Autodesk Inventor part; units mm, degrees
ref_plane "YZ Plane" through (0, 0, 0) normal (1, 0, 0) x (0, 1, 0)
ref_plane "XZ Plane" through (0, 0, 0) normal (0, 1, 0) x (-1, 0, 0)
ref_plane "XY Plane" through (0, 0, 0) normal (0, 0, 1) x (1, 0, 0)
sketch "Sketch1" plane through (0, 0, 0) normal (0, 0, 1) x (1, 0, 0)
  line L0 (-4.5718, -2.6632) -> (-7.5718, -2.6632)
  line L1 (-7.5718, -2.6632) -> (-7.5718, -10.8132)
  line L2 (-7.5718, -10.8132) -> (-4.5718, -10.8132)
  line L3 (-4.5718, -10.8132) -> (-4.5718, -2.6632)
  dimension "d1" = 8.15
  dimension "d2" = 3
revolve "Shoulder" add sketch "Sketch1" angle 360 about axis through (-4.5718, -10.8132, 0) along (0, 1, 0)
sketch "Sketch2" plane through (-4.5718, -2.6632, 0) normal (0, 1, 0) x (1, 0, 0)
  circle A0 centre (0, 0) radius 3
  circle A1 centre (0, 0) radius 2.76
  dimension "d3" = 5.52
extrude "Shoulder_neck" add sketch "Sketch2" along normal blind 1.85 contours A1
sketch "Sketch3" plane through (-4.5718, -0.8132, 0) normal (0, 1, 0) x (1, 0, 0)
  circle A0 centre (0, 0) radius 2.76
  circle A1 centre (0, 0) radius 5.075
  dimension "d6" = 10.15
extrude "Head" add sketch "Sketch3" along normal blind 4.5 contours A0 | A1
sketch "Sketch4" plane through (-4.5718, -10.8132, 0) normal (0, -1, 0) x (1, 0, 0)
  circle A0 centre (0, 0) radius 3
  circle A1 centre (0, 0) radius 1.89
  dimension "d9" = 3.78
extrude "Thread_neck" add sketch "Sketch4" along normal blind 1.8 contours A1
sketch "Sketch5" plane through (-4.5718, -12.6132, 0) normal (0, -1, 0) x (1, 0, 0)
  circle A0 centre (0, 0) radius 1.89
  circle A1 centre (0, 0) radius 2.5
  dimension "d12" = 5
extrude "Thread_shoulder" add sketch "Sketch5" along normal blind 7.7 contours A0 | A1
sketch "Sketch6" plane through (-4.5718, 3.6868, 0) normal (0, 1, 0) x (1, 0, 0)
  circle A0 centre (0, 0) radius 5.075
  circle A1 centre (0, 0) radius 1.5 construction
  line L0 (-1.5, 0.866) -> (-1.5, -0.866)
  line L1 (-1.5, -0.866) -> (0, -1.7321)
  line L2 (0, -1.7321) -> (1.5, -0.866)
  line L3 (1.5, -0.866) -> (1.5, 0.866)
  line L4 (1.5, 0.866) -> (0, 1.7321)
  line L5 (0, 1.7321) -> (-1.5, 0.866)
  dimension "d15" = 3
extrude "Hex" cut sketch "Sketch6" against normal blind 2.4 contours L5 L4 L3 L2 L1 L0
chamfer "Chamfer1" distance 0.24 angle 30 1 edges at (-1.5718, -2.6632, 0) measured on face at (-7.436, -2.6632, -0.4595)
fillet "Fillet1" radius 0.4 1 edges at (-7.3318, -0.8132, 0)
chamfer "Chamfer2" distance 0.3 angle 30 1 edges at (-9.6468, 3.6868, 0) measured on face at (0.4867, 2.1868, 0.4084)
chamfer "Chamfer3" distance 0.4 angle 30 1 edges at (-7.0718, -20.3132, 0) measured on face at (-3.3106, -20.3132, -0.6619)
fillet "Fillet2" radius 0.6 1 edges at (-6.4618, -10.8132, 0)
chamfer "Chamfer7" distance 0.61 angle 30 1 edges at (-7.0718, -12.6132, 0) measured on face at (-2.3177, -12.6132, -0.3502)
thread "Thread"
equation "\"d1\" = Shoulder_length - Shoulder_neck_length"
equation "\"d2\" = 0.5 * Shoulder_diameter"
equation "\"d3\" = Shoulder_neck_dia"
equation "\"d4\" = Shoulder_neck_length"
equation "\"d6\" = Head_diameter"
equation "\"d7\" = Head_height"
equation "\"d9\" = Thread_neck_dia"
equation "\"d10\" = Thread_neck_length"
equation "\"d12\" = Thread_diameter"
equation "\"d13\" = Thread_length - Thread_neck_length"
equation "\"d15\" = Hex_size"
equation "\"d16\" = Hex_length"
equation "\"d18\" = -0.5 * Shoulder_neck_dia + 0.5 * Shoulder_diameter"
equation "\"d64\" = -0.5 * Shoulder_neck_dia + 0.5 * Shoulder_diameter"
equation "\"d21\" = 0.1 * Hex_size"
equation "\"d65\" = 0.1 * Hex_size"
equation "\"d23\" = 0.5 * Thread_pitch"
equation "\"d66\" = 0.5 * Thread_pitch"
equation "\"d25\" = Thread_neck_radius"
equation "\"d60\" = -0.5 * Thread_neck_dia + 0.5 * Thread_diameter"
equation "\"d67\" = -0.5 * Thread_neck_dia + 0.5 * Thread_diameter"
equation "\"Shoulder_diameter\" = 6"
equation "\"Shoulder_length\" = 10"
equation "\"Shoulder_neck_dia\" = 5.52"
equation "\"Thread_diameter\" = 5"
equation "\"Thread_length\" = 9.5"
equation "\"Head_diameter\" = 10.15"
equation "\"Head_height\" = 4.5"
equation "\"Thread_neck_dia\" = 3.78"
equation "\"Hex_size\" = 3"
equation "\"Hex_length\" = 2.4"
equation "\"Thread_pitch\" = 0.8"
equation "\"Shoulder_neck_length\" = 1.85"
equation "\"Thread_neck_length\" = 1.8"
equation "\"Thread_neck_radius\" = 0.6"
properties part number "SCREW, SHOULDER, P, 12.9,  M6X10MM" material "Steel, High Strength Low Alloy"
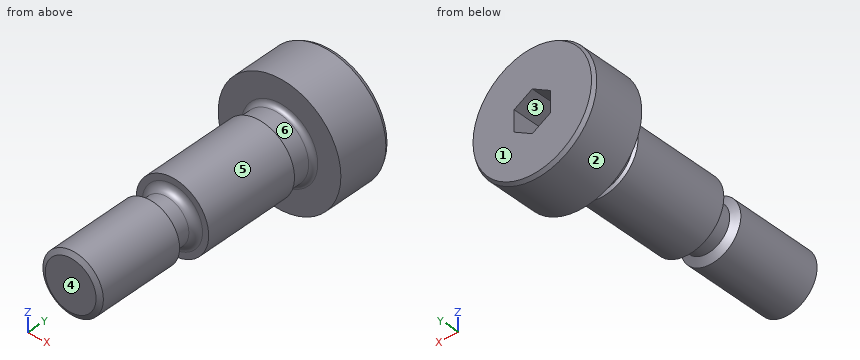
CAD build for the part. Positions are in the model's coordinates, mm. Face numbers are marked on the shaded views. A direction names the side the tool comes from. Coordinates: 2 decimals unless noted, no trailing zeros. Order: outer loops, then holes, each group sorted by start corner. A loop starts at its lowest first (then second) coordinate and runs counter-clockwise, first axis right, second up.
Item 1: Two-plate mould, pull along Z, no slides. Class the marked faces 1, 2 and 3: +Z half, -Z half, draft (parallel to the pull), parting line (faces both ways), or undercut.
Check sheet entries:
face 1: draft
face 2: parting line
face 3: undercut
Item 2: Pin check, flat tips, straight feed: pin 1 Ø6 at (x, z) = (-5, 1) entering from +Y; pin 2 Ø2 at (y, z) = (-11, 0.5) entering from -X; pin 3 Ø1.5 at (y, z) = (-9.5, -2) entering from +X; pin 4 Ø5 at (x, z) = (-1, -3) entering from -Y. Stop position of each tip, or through.
Check sheet entries:
pin 1: stops at y = 3.69
pin 2: stops at x = -7.57
pin 3: stops at x = -1.84
pin 4: stops at y = -20.28
Item 3: 3-axis set-ups, long thin cutter, end or side, ignore diameter. For the marked faces 4, 5 and 6: which of +Z, -Z, +X, -X, +Y, -Y reach the whole face in a straight line?
Check sheet entries:
face 4: +Z, -Z, +X, -X, -Y
face 5: -Y
face 6: none
Item 4: Drill centre lines: L1, parallel to Y at x = -7, z = 1.25; L2, parallel to Y at x = -1, z = -3.25; L3, parallel to X at y = 1.75, z = 1. Where is each one in solid material? Low to high.
Check sheet entries:
L1: y = -10.81 to 3.69
L2: y = -0.81 to 3.69
L3: x = -9.55 to -5.84, -3.3 to 0.4
Item 5: Band-saw the part on B-B on y = -1.75. List the corners of the cut face in (x, z).
Check sheet entries:
outline: circle Ø5.52 at (-4.57, 0)
Item 6: Band-saw the part on A-A on y = 1.75. List the corners of the cut face in (x, z) (3 decimals), plus the area to 3 significant figures.
Check sheet entries:
outline: circle Ø10.15 at (-4.572, 0); hole (-6.072, -0.866) - (-4.572, -1.732) - (-3.072, -0.866) - (-3.072, 0.866) - (-4.572, 1.732) - (-6.072, 0.866) - close
area: 73.1 mm2
